Verification items for the finished model (mm, model axes). A direction names the side the tool comes from. Give positions to 0.01 mm unless a question says otherwise; leave off trailing zeros. Loops run counter-clockwise (first coordinate to the right, second up) from the corner with the lowest first, then second, coordinate; pieces in that order, holes last. Notation, with made-up numbers: (-37, 67) -> (22, 67) arc R6 cw to (22, 77) -> close; hole circle Ø4 at (85, 65). An arc over 180 degrees is marked (long way). Answer in a Markdown table with one row per item. Add a question column.
Q1. Material ranges on probe 1 along X at (y, z) = (3.75, -5.5); probe 2 along X at (y, z) = (7.25, 2.5); probe 3 along X at (y, z) = (4.75, 18), recorded low to high.
Q2. Set-up check for faces 5 (the face through (-20.337, 3.845, 21.093)), 6 (the face through (-25, 7, 4)), 7 (the face through (-22, 0.8, 8)), 8 (the face through (-33, 4, 14.891)): record each of +Z, -Z, +X, -X, +Y, -Y from which the full face is reachable in a straight line by a thin tool's end or side.
Q3. Section check C-C on y = 3.5. Enter the section's corners in (x, z), and give its area (3 significant figures).
Q4. Section check A-A on x = -29.25. Enter the section's corners in (y, z).
Q5. Section check D-D on x = -23.5. Give the number of separate pieces and of enclosed holes in the cut face, and give its area (3 significant figures).
Q6. Release check for a two-part mould opening along Z. For faces 1 (the face through (-42.66, 3.85, 18.62)), 2 (the face through (-23.03, 3.85, -17.27)), 3 (the face through (-20.04, 7.41, 1.54)), 4 (the face through (-40.78, 3.86, 16.92)) record: pulls with the +Z half, pulls with the -Z half, needs draft (parallel to the pull), parting line crosses it, or undercut.
Q7. Gauge pin test, flat ends, axial feed: P1, Ø5.5, axis at x = -22.95, z = -5.58, coming from the +Y side; P2, Ø1.5, axis at y = 5, z = 3.5, coming from the -X side; P3, Ø1.5, axis at x = -25.5, z = -10, coming from the -Y side; P4, Ø1.8, axis at x = -21.5, z = -6.5, coming from the -Y side. Record the tip position at first contact, or that the pin passes through.
Q8. Section check B-B on z = 10. Enter the section's corners in (x, y).
```python
from build123d import *

# Parameters (mm, degrees)
SKETCH1_R           = 2.4
BOSS_EXTRUDE1_DEPTH = 7.8
SKETCH2_R           = 3.05
CUT_EXTRUDE1_DEPTH  = 0.8
SKETCH3_R           = 3.05
CUT_EXTRUDE2_DEPTH  = 0.8


with BuildPart() as part:
    # Sketch1 → Boss-Extrude1 (new body)
    with BuildSketch(Plane(origin=(0, 0, 0), x_dir=(1, 0, 0), z_dir=(0, 1, 0))):
        with BuildLine():
            Line((-39.012427485, -14.890555083), (-26.596473565, -14.89055472))
            Line((-26.596473565, -14.89055472), (-26.596474399, 13.619444917))
            ThreePointArc((-26.596474399, 13.619444917), (-22.946475341, 17.269443976), (-19.296476282, 13.619444917))
            Line((-19.296476282, 13.619444917), (-19.296475341, -18.540555083))
            ThreePointArc((-19.296475341, -18.540555083), (-20.365535589, -21.121494834), (-22.946475341, -22.190555083))
            Line((-22.946475341, -22.190555083), (-39.012427485, -22.190555083))
            ThreePointArc((-39.012427485, -22.190555083), (-42.662427485, -18.540555083), (-39.012427485, -14.890555083))
        make_face()
        with Locations((-39.012427485, -18.540555083)):
            Circle(SKETCH1_R, mode=Mode.SUBTRACT)
        with Locations((-30.972427485, -18.540555083)):
            Circle(SKETCH1_R, mode=Mode.SUBTRACT)
        with Locations((-22.946475341, -18.540555083)):
            Circle(SKETCH1_R, mode=Mode.SUBTRACT)
        with Locations((-22.946475341, 13.619444917)):
            Circle(SKETCH1_R, mode=Mode.SUBTRACT)
        with Locations((-22.946475341, 5.579444917)):
            Circle(SKETCH1_R, mode=Mode.SUBTRACT)
        with Locations((-22.946475341, -2.460555083)):
            Circle(SKETCH1_R, mode=Mode.SUBTRACT)
        with Locations((-22.946475341, -10.500555083)):
            Circle(SKETCH1_R, mode=Mode.SUBTRACT)
    extrude(amount=BOSS_EXTRUDE1_DEPTH)

    # Sketch2 → Cut-Extrude1 (cut)
    with BuildSketch(Plane(origin=(0, 7.8, 0), x_dir=(1, 0, 0), z_dir=(0, 1, 0))):
        with Locations((-39.012427485, -18.540555083)):
            Circle(SKETCH2_R)
        with Locations((-30.972427485, -18.540555083)):
            Circle(SKETCH2_R)
        with Locations((-22.946475341, -18.540555083)):
            Circle(SKETCH2_R)
        with Locations((-22.946475341, -10.500555083)):
            Circle(SKETCH2_R)
        with Locations((-22.946475341, -2.460555083)):
            Circle(SKETCH2_R)
        with Locations((-22.946475341, 5.579444917)):
            Circle(SKETCH2_R)
        with Locations((-22.946475341, 13.619444917)):
            Circle(SKETCH2_R)
    extrude(amount=-CUT_EXTRUDE1_DEPTH, mode=Mode.SUBTRACT)

    # Sketch3 → Cut-Extrude2 (cut)
    with BuildSketch(Plane.XZ):
        with Locations((-30.972427485, 18.540555083)):
            Circle(SKETCH3_R)
        with Locations((-39.012427485, 18.540555083)):
            Circle(SKETCH3_R)
        with Locations((-22.946475341, 18.540555083)):
            Circle(SKETCH3_R)
        with Locations((-22.946475341, 10.500555083)):
            Circle(SKETCH3_R)
        with Locations((-22.946475341, 2.460555083)):
            Circle(SKETCH3_R)
        with Locations((-22.946475341, -5.579444917)):
            Circle(SKETCH3_R)
        with Locations((-22.946475341, -13.619444917)):
            Circle(SKETCH3_R)
    extrude(amount=-CUT_EXTRUDE2_DEPTH, mode=Mode.SUBTRACT)


solid = part.part
```
Taken from the geometry:
| question | item | result |
|---|---|---|
| 1 | probe 1 | x = -26.6 to -25.35, -20.55 to -19.3 |
| 1 | probe 2 | x = -26.6 to -26, -19.9 to -19.3 |
| 1 | probe 3 | x = -42.62 to -41.35, -36.67 to -33.31, -28.63 to -25.28, -20.61 to -19.3 |
| 2 | face 5 | +Z, +X, +Y, -Y |
| 2 | face 6 | +Y |
| 2 | face 7 | -Y |
| 2 | face 8 | -Z, -X, +Y, -Y |
| 3 | outline | (-39.01, 14.89) -> (-26.6, 14.89) -> (-26.6, -13.62) arc R3.65 ccw to (-19.3, -13.62) -> (-19.3, 18.54) arc R3.65 ccw to (-22.95, 22.19) -> (-39.01, 22.19) arc R3.65 ccw to start; hole circle Ø4.8 at (-39.01, 18.54); hole circle Ø4.8 at (-30.97, 18.54); hole circle Ø4.8 at (-22.95, -13.62); hole circle Ø4.8 at (-22.95, -5.58); hole circle Ø4.8 at (-22.95, 2.46); hole circle Ø4.8 at (-22.95, 10.5); hole circle Ø4.8 at (-22.95, 18.54) |
| 3 | area | 264 mm² |
| 4 | outline | (0, 14.89) -> (7.8, 14.89) -> (7.8, 16.02) -> (7, 16.02) -> (7, 16.87) -> (0.8, 16.87) -> (0.8, 16.02) -> (0, 16.02) -> close; (0, 21.06) -> (0.8, 21.06) -> (0.8, 20.21) -> (7, 20.21) -> (7, 21.06) -> (7.8, 21.06) -> (7.8, 22.19) -> (0, 22.19) -> close |
| 5 | separate pieces | 6 |
| 5 | enclosed holes | 0 |
| 5 | area | 115 mm² |
| 6 | face 1 | parting line crosses it |
| 6 | face 2 | pulls with the -Z half |
| 6 | face 3 | undercut |
| 6 | face 4 | undercut |
| 7 | P1 | stops at y = 7 |
| 7 | P2 | stops at x = -26.6 |
| 7 | P3 | stops at y = 0 |
| 7 | P4 | stops at y = 0.8 |
| 8 | outline | (-26.6, 0) -> (-25.96, 0) -> (-25.96, 0.8) -> (-25.29, 0.8) -> (-25.29, 7) -> (-25.96, 7) -> (-25.96, 7.8) -> (-26.6, 7.8) -> close; (-20.6, 0.8) -> (-19.94, 0.8) -> (-19.94, 0) -> (-19.3, 0) -> (-19.3, 7.8) -> (-19.94, 7.8) -> (-19.94, 7) -> (-20.6, 7) -> close |
